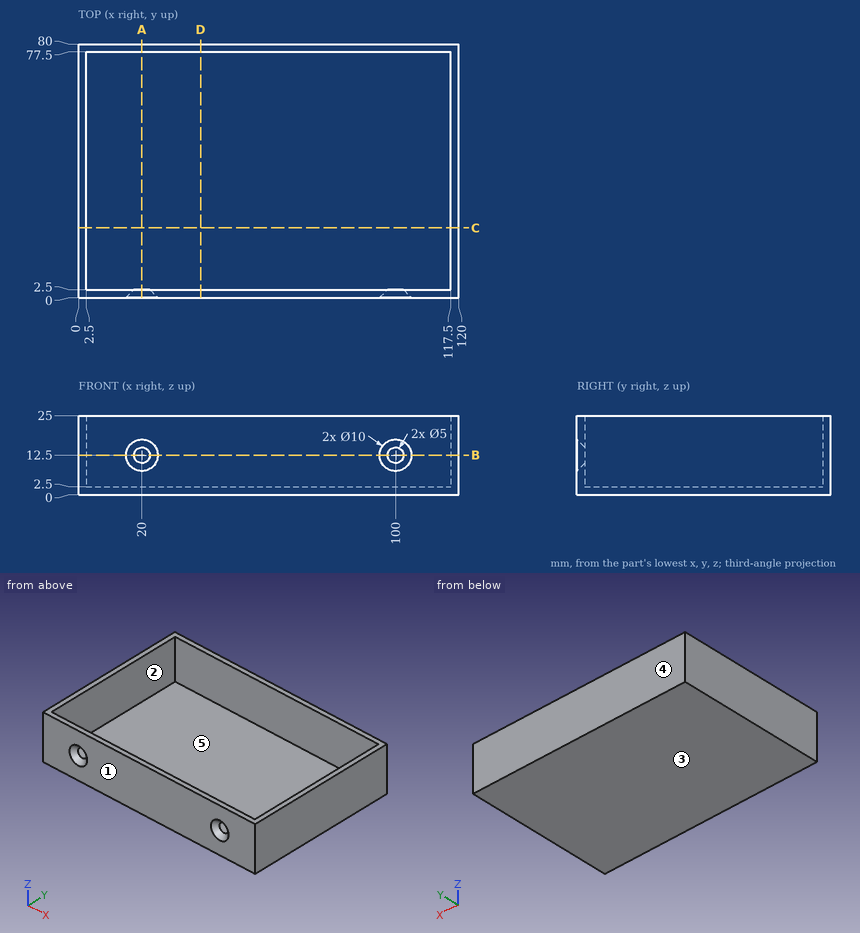
Study the drawing (mm; zero at the part's minimum x, y, z) and answer. A direction names the side the tool comes from. Round coordinates to 2 decimals unless told otherwise and drop trailing zeros. Loops run counter-clockwise (first coordinate to the right, second up) from the corner with the lowest first, then second, coordinate; pieces in that order, holes last. Notation, with made-up numbers: (70.5, 73.25) -> (125.5, 73.25) arc R21 ccw to (125.5, 83.25) -> close; hole circle Ø5 at (-30, 17). An arc over 180 degrees is marked (long way). Write each question's results on one line, items separated by ' | '. Start each with the question number.
1. Given pin 1 Ø1.5 at (x, y) = (15.5, 35) entering from +Z, flat-ended and moving along its own axis, determine where the tip first touches the part or whether it passes through.
2. For a pull along Y with two mould halves and no side action, classify the marked faces 3, 4 and 5 as +Y half, -Y half, draft (parallel to the pull), parting line (faces both ways), or undercut.
3. Section A-A (x = 20) is taken. Determine the outline of the cut face in (y, z).
4. A tool of negligible diameter and unlimited length cuts with its end or side. For the marked faces 1 and 2, from which of +Z, -Z, +X, -X, +Y, -Y can it reach the whole face along a straight path? Write none if from no direction.
5. Section B-B (z = 12.5) is taken. Determine the outline of the cut face in (x, y), plus the area to 4 significant figures.
6. Section D-D (x = 38.5) is taken. Determine the outline of the cut face in (y, z), plus the area to 4 significant figures.
7. Section C-C (y = 22) is taken. Determine the outline of the cut face in (x, z).
8. Find the intervals of material crossed by probe 1 along X at (y, z) = (16, 23.75); probe 2 along Y at (x, z) = (103, 20); probe 3 along Z at (x, y) = (60, 46), in increasing order. Write a range as from..to.
Evaluation:
1) pin 1: stops at z = 2.5
2) face 3: draft | face 4: +Y half | face 5: undercut
3) outline: (0, 0) -> (80, 0) -> (80, 25) -> (77.5, 25) -> (77.5, 2.5) -> (2.5, 2.5) -> (2.5, 10) -> (0, 7.5) -> close; (0, 17.5) -> (2.5, 15) -> (2.5, 25) -> (0, 25) -> close
4) face 1: +Z, -Z, +X, -X, -Y | face 2: +Z
5) outline: (0, 0) -> (15, 0) -> (17.5, 2.5) -> (2.5, 2.5) -> (2.5, 77.5) -> (117.5, 77.5) -> (117.5, 2.5) -> (102.5, 2.5) -> (105, 0) -> (120, 0) -> (120, 80) -> (0, 80) -> close; (22.5, 2.5) -> (25, 0) -> (95, 0) -> (97.5, 2.5) -> close | area: 937.5 mm2
6) outline: (0, 0) -> (80, 0) -> (80, 25) -> (77.5, 25) -> (77.5, 2.5) -> (2.5, 2.5) -> (2.5, 25) -> (0, 25) -> close | area: 312.5 mm2
7) outline: (0, 0) -> (120, 0) -> (120, 25) -> (117.5, 25) -> (117.5, 2.5) -> (2.5, 2.5) -> (2.5, 25) -> (0, 25) -> close
8) probe 1: x = 0..2.5, 117.5..120 | probe 2: y = 0..2.5, 77.5..80 | probe 3: z = 0..2.5
